```python
from build123d import *

# Parameters (mm, degrees)
SKETCH_5_W          = 80
SKETCH_5_H          = 60
EXTRUDE_5_DEPTH     = 10
EXTRUDE_6_DEPTH     = 10
EXTRUDE_9_DEPTH     = 6
EXTRUDE_10_DEPTH    = 6
SKETCH_11_R         = 10
CUT_EXTRUDE_1_DEPTH = 101.498756211
SKETCH_13_R         = 5
CUT_EXTRUDE_3_DEPTH = 101.498756211


with BuildPart() as part:
    # 草图5 → 凸台-拉伸5 (new body)
    with BuildSketch(Plane(origin=(0, 0, 0), x_dir=(1, 0, 0), z_dir=(0, 1, 0))):
        with Locations((0, -30)):
            Rectangle(SKETCH_5_W, SKETCH_5_H)
    extrude(amount=EXTRUDE_5_DEPTH)

    # 草图6 → 凸台-拉伸6 (add)
    with BuildSketch(Plane.XY):
        with BuildLine():
            Line((-40, 0), (40, 0))
            Line((40, 0), (40, 60))
            ThreePointArc((40, 60), (37.071067812, 67.071067812), (30, 70))
            Line((30, 70), (-30, 70))
            ThreePointArc((-30, 70), (-37.071067812, 67.071067812), (-40, 60))
            Line((-40, 60), (-40, 0))
        make_face()
    extrude(amount=EXTRUDE_6_DEPTH)

    # 草图9 → 凸台-拉伸9 (add)
    with BuildSketch(Plane(origin=(-40, 0, 0), x_dir=(0, 0, -1), z_dir=(1, 0, 0))):
        Polygon((-10, 10), (-50, 10), (-10, 50), align=None)
    extrude(amount=EXTRUDE_9_DEPTH)

    # 草图10 → 凸台-拉伸10 (add)
    with BuildSketch(Plane(origin=(34, 0, 0), x_dir=(0, 0, -1), z_dir=(1, 0, 0))):
        Polygon((-10, 10), (-50, 10), (-10, 50), align=None)
    extrude(amount=EXTRUDE_10_DEPTH)

    # 草图11 → 切除-拉伸1 (cut, through all)
    with BuildSketch(Plane.XY):
        with Locations((0, 45)):
            Circle(SKETCH_11_R)
    extrude(amount=CUT_EXTRUDE_1_DEPTH, mode=Mode.SUBTRACT)

    # 草图13 → 切除-拉伸3 (cut, through all)
    with BuildSketch(Plane(origin=(0, 0, 0), x_dir=(1, 0, 0), z_dir=(0, 1, 0))):
        with Locations(Location((-28, -42, 0), (0, 0, 90))):
            Circle(SKETCH_13_R)
        with Locations(Location((28, -42, 0), (0, 0, 90))):
            Circle(SKETCH_13_R)
    extrude(amount=CUT_EXTRUDE_3_DEPTH, mode=Mode.SUBTRACT)


solid = part.part
```
Model file for the job. Use its own axes, mm. A direction names the side the tool comes from. Coordinates: 2 decimals unless noted, no trailing zeros. Loops run counter-clockwise (first coordinate to the right, second up) from the corner with the lowest first, then second, coordinate; pieces in that order, holes last. Notation, with made-up numbers: (-13.75, 70.25) - (-4.75, 70.25) arc R18 ccw to (-4.75, 76.25) - close; hole circle Ø6 at (36, 40.25). An arc over 180 degrees is marked (long way). Write item = value, one per line. Start each with the question number.
Item 1: Saw through at A-A, the plane z = 42. List the corners of the cut face in (x, y), then the cut area to 3 significant figures.
Item 2: Pull direction X, two halves, no side cores. Call faces 1 (the face through (-37, 30, 30)), 2 (the face through (-36.99, 67.15, 4.93)), 3 (the face through (-25, 5, 46)), 4 (the face through (40, 24, 16)): +X half, -X half, draft (parallel to the pull), parting line (faces both ways), or undercut.
Item 3: 3-axis set-ups, long thin cutter, end or side, ignore diameter. For faces 5 (the face through (-1, 10, 35)), 6 (the face through (37, 30, 30)): which of +Z, -Z, +X, -X, +Y, -Y reach the whole face in a straight line?
Item 4: Drop flat-ended pins along their axis: pin 1 Ø1 at (x, z) = (-29, 36.5) entering from +Y; pin 2 Ø4 at (x, y) = (30.5, 7.5) entering from -Z. Give the stop position or say it passes through.
Item 5: Saw through at C-C, the plane y = 53. List the corners of the cut face in (x, z), then the cut area to 3 significant figures.
Item 6: Saw through at D-D, the plane z = 20.5. List the corners of the cut face in (x, y).
Item 7: Wall check: probe 1 along X at (y, z) = (4, 42); probe 2 along X at (y, z) = (45, 8); probe 3 along X at (y, z) = (14, 42.5). Give the ranges that are in metal, low to high. Write a range as [from, to].
Item 8: Saw through at B-B, the plane x = 28. List the corners of the cut face in (y, z), then the cut area to 3 significant figures.
Answers:
q1.outline = (-40, 0) - (-33, 0) - (-33, 10) - (-34, 10) - (-34, 18) - (-40, 18) - close; (-23, 0) - (23, 0) - (23, 10) - (-23, 10) - close; (33, 0) - (40, 0) - (40, 18) - (34, 18) - (34, 10) - (33, 10) - close
q1.area = 696 mm2
q2.face_1 = draft
q2.face_2 = -X half
q2.face_3 = undercut
q2.face_4 = +X half
q3.face_5 = +Z, +Y
q3.face_6 = +Z, +X, -X, +Y
q4.pin_1 = 10
q4.pin_2 = 0
q5.outline = (-40, 0) - (-6, 0) - (-6, 10) - (-40, 10) - close; (6, 0) - (40, 0) - (40, 10) - (6, 10) - close
q5.area = 680 mm2
q6.outline = (-40, 0) - (40, 0) - (40, 39.5) - (34, 39.5) - (34, 10) - (-34, 10) - (-34, 39.5) - (-40, 39.5) - close
q7.probe_1 = [-40, -33], [-23, 23], [33, 40]
q7.probe_2 = [-40, -10], [10, 40]
q7.probe_3 = [-40, -34], [34, 40]
q8.outline = (0, 0) - (70, 0) - (70, 10) - (10, 10) - (10, 37) - (0, 37) - close; (0, 47) - (10, 47) - (10, 60) - (0, 60) - close
q8.area = 1,100 mm2
